from build123d import *

# Parameters (mm, degrees)
SKETCH2_R          = 5
SKETCH2_W          = 5.5
SKETCH2_H          = 5.5
CUT_EXTRUDE1_DEPTH = 6


with BuildPart() as part:
    # Sketch1 → Revolve1 (revolve)
    with BuildSketch(Plane.XY, mode=Mode.PRIVATE) as revolve1_sk:
        Polygon((0, 0), (0, 3.9), (1.678312164, 3.9), (2.4, 2.65), (2.4, 0), align=None)
    revolve(revolve1_sk.sketch.rotate(Axis((2.4, 0, 0), (-1, 0, 0)), 270), axis=Axis((2.4, 0, 0), (-1, 0, 0)))

    # Sketch2 → Cut-Extrude1 (cut)
    with BuildSketch(Plane(origin=(0, 0, 0), x_dir=(0, 0, -1), z_dir=(1, 0, 0))):
        Circle(SKETCH2_R)
        Rectangle(SKETCH2_W, SKETCH2_H, mode=Mode.SUBTRACT)
    extrude(amount=CUT_EXTRUDE1_DEPTH, mode=Mode.SUBTRACT)

    # Sketch3 → Cut-Revolve1 (revolve, cut)
    with BuildSketch(Plane.XY, mode=Mode.PRIVATE) as cut_revolve1_sk:
        Polygon((0, 0), (0, 1.5), (0.2705, 1.2295), (2.1295, 1.2295), (2.4, 1.5), (2.4, 0), align=None)
    revolve(cut_revolve1_sk.sketch.rotate(Axis((2.4, 0, 0), (-1, 0, 0)), 270), axis=Axis((2.4, 0, 0), (-1, 0, 0)), mode=Mode.SUBTRACT)


solid = part.part
Source: CAD feature listing. Evaluate the final solid. Frame: model axes, mm. Round coordinates to 2 decimals unless told otherwise and drop trailing zeros. Loops run counter-clockwise (first coordinate to the right, second up) from the corner with the lowest first, then second, coordinate; pieces in that order, holes last. Notation, with made-up numbers: (42, 82) -> (90, 82) arc R27 cw to (90, 102) -> close; hole circle Ø2 at (-40, -22.75). An arc over 180 degrees is marked (long way). Answer as a JSON object with one key per item and string values. Group by question number.
Q1. Section query A-A (z = 0). Output: boundary loops of the cut face in (x, y).
Q2. Mould query, pull axis Z, two halves, no side actions, for faces 1 (the flat face through (1, 2.75, 0)), 2 (the flat face through (1, 0, -2.75)), 3 (the flat face through (1, 0, 2.75)), 4 (the cylindrical face through (1.21, -1.2, -0.27)). Classes: pulls with the +Z half, pulls with the -Z half, needs draft (parallel to the pull), parting line crosses it, or undercut.
Q3. Ray query, line 1 (Y direction, x = 1.2, z = 0); line 2 (Z direction, x = 1.95, y = -0.65); line 3 (Z direction, x = 0.6, y = 0.5). Return the intervals inside material, ascending. Write a range as from..to.
Q4. Contact query for a flat-ended pin moving along its axis: P1, Ø2, axis at y = 0, z = 0, coming from the +X side. Output: stop coordinate, or through.
Q5. Section query B-B (x = 1.6). Output: boundary loops of the cut face in (y, z), plus the area to 3 significant figures.
Q6. Section query C-C (x = 1.95). Output: boundary loops of the cut face in (y, z), plus the area to 3 significant figures.
Completed:
{
 "1": {"outline": "(0, -2.75) -> (2.34, -2.75) -> (2.4, -2.65) -> (2.4, -1.5) -> (2.13, -1.23) -> (0.27, -1.23) -> (0, -1.5) -> close; (0, 1.5) -> (0.27, 1.23) -> (2.13, 1.23) -> (2.4, 1.5) -> (2.4, 2.65) -> (2.34, 2.75) -> (0, 2.75) -> close"},
 "2": {"face 1": "needs draft", "face 2": "pulls with the -Z half", "face 3": "pulls with the +Z half", "face 4": "undercut"},
 "3": {"line 1": "-2.75..-1.23, 1.23..2.75", "line 2": "-2.75..-1.04, 1.04..2.75", "line 3": "-2.75..-1.12, 1.12..2.75"},
 "4": {"P1": "through"},
 "5": {"outline": "(-2.75, -2.75) -> (2.75, -2.75) -> (2.75, 2.75) -> (-2.75, 2.75) -> close; hole circle Ø2.46 at (0, 0)", "area": "25.5 mm²"},
 "6": {"outline": "(-2.75, -2.05) arc R3.43 ccw to (-2.05, -2.75) -> (2.05, -2.75) arc R3.43 ccw to (2.75, -2.05) -> (2.75, 2.05) arc R3.43 ccw to (2.05, 2.75) -> (-2.05, 2.75) arc R3.43 ccw to (-2.75, 2.05) -> close; hole circle Ø2.46 at (0, 0)", "area": "24.6 mm²"}
}
